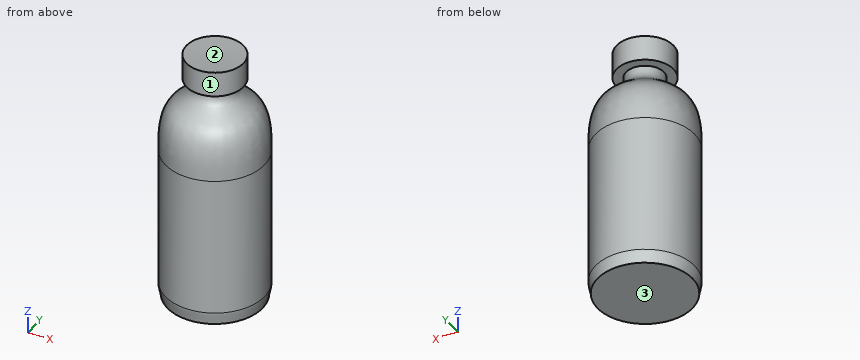
```python
from build123d import *


with BuildPart() as f1:
    # F0 (on Front) → F1 (revolve)
    with BuildSketch(Plane.XZ):
        with BuildLine():
            Line((-37.4588370323, 59.732876718), (-37.4588370323, 48.8092340529))
            Line((-37.4588370323, 48.8092340529), (-37.4588370323, -45.6943430106))
            add(Edge.make_bspline(
                [(-37.4588370323, -45.6943430106), (-37.6298800111, -48.9646402564), (-35.7483886182, -52.1555552913), (-35.919431597, -55.4258525372)],
                knots=[0, 0, 0, 0, 9.852514743, 9.852514743, 9.852514743, 9.852514743], degree=3))
            Line((-35.919431597, -55.4258525372), (0, -55.4258525372))
            Line((0, -55.4258525372), (0, 126.7814934254))
            Line((0, 126.7814934254), (0, 135.206669569))
            Line((0, 135.206669569), (-21.5448252857, 135.9217166901))
            Line((-21.5448252857, 135.9217166901), (-21.5448252857, 116.9883906841))
            Line((-21.5448252857, 116.9883906841), (-14.3632190302, 116.9883906841))
            add(Edge.make_bspline(
                [(-37.4588370323, 59.732876718), (-37.8051019347, 75.656499795), (-35.7428372279, 95.5439069808), (-14.945244298, 104.3960584298), (-14.0862612605, 112.3647683936), (-14.3632190302, 116.9883906841)],
                knots=[0, 0, 0, 0, 0.4379829854, 0.7509225673, 1, 1, 1, 1], degree=3))
        make_face()
    revolve(axis=Axis((0, 0, 35.6778204441), (0, 0, -1)))


solid = f1.part
```
Design review of the part built by this model. Coordinates are the model's own, in mm. Face numbers are marked on the shaded views. Coordinates: 2 decimals unless noted, no trailing zeros. Loops run counter-clockwise (first coordinate to the right, second up) from the corner with the lowest first, then second, coordinate; pieces in that order, holes last.
Q1. The part is to be moulded in two halves that separate along Y. For the marked faces 1, 2 and 3, say which applies: +Y half, -Y half, draft (parallel to the pull), parting line (faces both ways), or undercut.
Reported:
face 1: parting line
face 2: undercut
face 3: draft
Q2. To check wall thickness, follow line 1 (Z direction, x = -1, y = -0.5); line 2 (Z direction, x = -0.5, y = 31); line 3 (Z direction, x = 8.5, y = -14). State the ranges of each line that lie inside material, in increasing order.
Reported:
line 1: z = -55.43 to 135.24
line 2: z = -55.43 to 94.08
line 3: z = -55.43 to 106.66, 116.99 to 135.75
Q3. For pin 1 (8 mm diameter, centred on x = 11, y = -30, fed in from +Z); pin 2 (4 mm diameter, centred on y = -3.5, z = 19.5, fed in from -X); pin 3 (2 mm diameter, centred on x = 7.5, z = 32, fed in from +Y), all flat-tipped, find the tip position at first contact; note any pin that passes through.
Reported:
pin 1: stops at z = 97.24
pin 2: stops at x = -37.43
pin 3: stops at y = 36.89
Q4. We need section A-A on z = 38.5. State the section outline as (x, y) points, and give its area (3 significant figures).
Reported:
outline: circle Ø74.92 at (0, 0)
area: 4,410 mm2
